```python
from build123d import *

# Parameters (mm, degrees)
SKETCH1_R                  = 96.35000288
BOSS_EXTRUDE1_DEPTH        = 6
SKETCH2_W                  = 2.86385
SKETCH2_H                  = 77.133562268
SKETCH2_W_2                = 77.133562268
SKETCH2_H_2                = 2.86385
CUT_EXTRUDE1_DEPTH         = 137.391517735
SKETCH3_W                  = 3.227804403
SKETCH3_H                  = 5
BOSS_EXTRUDE2_DEPTH        = 6
FILLET1_R                  = 9.525
F_6_4_6_4_DIAMETER_HOLE1_D = 6.4


with BuildPart() as part:
    # Sketch1 → Boss-Extrude1 (new body)
    with BuildSketch(Plane.XY):
        Circle(SKETCH1_R)
    extrude(amount=BOSS_EXTRUDE1_DEPTH)

    # Sketch2 → Cut-Extrude1 (cut, through all)
    with BuildSketch(Plane.XY.offset(6)):
        Polygon((6.122886862, 13.469001133), (44.689667996, 80.268625542), (47.169834848, 78.836700542), (8.603053714, 12.037076133), align=None)
        with Locations((0, 53.29272171)):
            Rectangle(SKETCH2_W, SKETCH2_H)
        Polygon((12.037076133, 8.603053714), (78.836700542, 47.169834848), (80.268625542, 44.689667996), (13.469001133, 6.122886862), align=None)
        with Locations((53.29272171, 0)):
            Rectangle(SKETCH2_W_2, SKETCH2_H_2)
        Polygon((13.469001133, -6.122886862), (80.268625542, -44.689667996), (78.836700542, -47.169834848), (12.037076133, -8.603053714), align=None)
        Polygon((8.603053714, -12.037076133), (47.169834848, -78.836700542), (44.689667996, -80.268625542), (6.122886862, -13.469001133), align=None)
        with Locations((0, -53.29272171)):
            Rectangle(SKETCH2_W, SKETCH2_H)
        Polygon((-6.122886862, -13.469001133), (-44.689667996, -80.268625542), (-47.169834848, -78.836700542), (-8.603053714, -12.037076133), align=None)
        Polygon((-12.037076133, -8.603053714), (-78.836700542, -47.169834848), (-80.268625542, -44.689667996), (-13.469001133, -6.122886862), align=None)
        with Locations((-53.29272171, 0)):
            Rectangle(SKETCH2_W_2, SKETCH2_H_2)
        Polygon((-13.469001133, 6.122886862), (-80.268625542, 44.689667996), (-78.836700542, 47.169834848), (-12.037076133, 8.603053714), align=None)
        Polygon((-8.603053714, 12.037076133), (-47.169834848, 78.836700542), (-44.689667996, 80.268625542), (-6.122886862, 13.469001133), align=None)
    extrude(amount=-CUT_EXTRUDE1_DEPTH, mode=Mode.SUBTRACT)

    # Sketch3 → Boss-Extrude2 (add)
    with BuildSketch(Plane.XY):
        with BuildLine():
            Line((203.2, 19), (94.45804918, 19))
            ThreePointArc((94.45804918, 19), (96.35000288, 0), (94.45804918, -19))
            Line((94.45804918, -19), (203.2, -19))
            Line((203.2, -19), (203.2, 19))
        make_face()
        with Locations((169.513902202, 10)):
            Rectangle(SKETCH3_W, SKETCH3_H, mode=Mode.SUBTRACT)
        with Locations((169.513902202, -10)):
            Rectangle(SKETCH3_W, SKETCH3_H, mode=Mode.SUBTRACT)
        with Locations((201.278368296, 10)):
            Rectangle(SKETCH3_W, SKETCH3_H, mode=Mode.SUBTRACT)
        with Locations((201.278368296, -10)):
            Rectangle(SKETCH3_W, SKETCH3_H, mode=Mode.SUBTRACT)
    extrude(amount=BOSS_EXTRUDE2_DEPTH)

    # Fillet1
    fillet1_edges = [part.edges().sort_by_distance(p)[0] for p in [
        (94.45804918, -19, 3),
        (94.45804918, 19, 3),
    ]]
    fillet(fillet1_edges, radius=FILLET1_R)

    # Ø6.4 (6.4) Diameter Hole1 (through all)
    with Locations(Plane.XY.offset(6)):
        with Locations((188.25889108, -10), (176.473462737, -10), (176.473462737, 10), (188.25889108, 10)):
            Hole(F_6_4_6_4_DIAMETER_HOLE1_D / 2)


solid = part.part
```
Can you work these out from the model? Positions are in its coordinate system, mm. A direction names the side the tool comes from. Round coordinates to 2 decimals unless told otherwise and drop trailing zeros. Order: outer loops, then holes, each group sorted by start corner. A loop starts at its lowest first (then second) coordinate and runs counter-clockwise, first axis right, second up.
(1) I'm going to push flat-ended pins straight in: pin 1 (1.8 mm diameter, centred on x = 44.5, z = 2, fed in from +Y); pin 2 (4 mm diameter, centred on x = 176.47, y = -10, fed in from -Z); pin 3 (1.5 mm diameter, centred on x = 168.5, z = 3.5, fed in from +Y); pin 4 (1.5 mm diameter, centred on x = -45, z = 0.5, fed in from -Y). Where does each tip first touch, or does it pass through?
Results are:
pin 1: stops at y = 85.92
pin 2: passes through
pin 3: stops at y = 19
pin 4: stops at y = -85.59
(2) If we section it at B-B (x = 70): Please give me the cut outline in (y, z), plus the area to 3 significant figures.
Results are:
outline: (-66.21, 0) - (-42.07, 0) - (-42.07, 6) - (-66.21, 6) - close; (-38.76, 0) - (-1.43, 0) - (-1.43, 6) - (-38.76, 6) - close; (1.43, 0) - (38.76, 0) - (38.76, 6) - (1.43, 6) - close; (42.07, 0) - (66.21, 0) - (66.21, 6) - (42.07, 6) - close
area: 738 mm2
(3) If we section it at A-A (y = -63.5): Please give me the cut outline in (x, z), plus the area to 3 significant figures.
Results are:
outline: (-72.46, 0) - (-38.32, 0) - (-38.32, 6) - (-72.46, 6) - close; (-35.01, 0) - (-1.43, 0) - (-1.43, 6) - (-35.01, 6) - close; (1.43, 0) - (35.01, 0) - (35.01, 6) - (1.43, 6) - close; (38.32, 0) - (72.46, 0) - (72.46, 6) - (38.32, 6) - close
area: 813 mm2
(4) On a 3-axis mill with a long thin cutter (end or side, diameter ignored), from which of +Z, -Z, +X, -X, +Y, -Y can I reach the whole of each face in a straight line? I mean faces 1 (the face through (203.2, 0, 3)), 2 (the face through (152, -19, 3)), 3 (the face through (25.68, -47.34, 3.04)). Say none if no direction works.
Results are:
face 1: +Z, -Z, +X, +Y, -Y
face 2: +Z, -Z, +X, -Y
face 3: +Z, -Z
(5) If I drill on L1, parallel to Y at x = 171, z = 2.25; L2, parallel to X at y = -84, z = 0.75; L3, parallel to Y at x = 37.5, z = 2.25, over which ranges is the centre line in solid material (lowest first)?
Results are:
L1: y = -19 to -12.5, -7.5 to 7.5, 12.5 to 19
L2: x = -47.19 to -1.43, 1.43 to 47.19
L3: y = -88.75 to -67.82, -62.09 to -23.3, -20 to -1.43, 1.43 to 20, 23.3 to 62.09, 67.82 to 88.75
(6) We'd pull the mould along X, two halves only. Please class faces 4 (the face through (18, 23, 6)), 5 (the face through (-28.156, -45.904, 3.042)), 6 (the face through (96.272, 20.885, 3.042)), 7 (the face through (27.616, -44.969, 3.042)): +X half, -X half, draft (parallel to the pull), parting line (faces both ways), or undercut.
Results are:
face 4: draft
face 5: undercut
face 6: +X half
face 7: undercut
(7) If we section it at C-C (x = 24): Please give me the cut outline in (y, z), plus the area to 3 significant figures.
Results are:
outline: (-93.31, 0) - (-44.43, 0) - (-44.43, 6) - (-93.31, 6) - close; (-38.71, 0) - (-15.51, 0) - (-15.51, 6) - (-38.71, 6) - close; (-12.2, 0) - (-1.43, 0) - (-1.43, 6) - (-12.2, 6) - close; (1.43, 0) - (12.2, 0) - (12.2, 6) - (1.43, 6) - close; (15.51, 0) - (38.71, 0) - (38.71, 6) - (15.51, 6) - close; (44.43, 0) - (93.31, 0) - (93.31, 6) - (44.43, 6) - close
area: 994 mm2
(8) If we section it at D-D (z = 4): Count the separate pieces of the cut face and the enclosed holes in it, plus the area to 3 significant figures.
Results are:
separate pieces: 1
enclosed holes: 20
area: 30,400 mm2
